from build123d import *

# Parameters (mm, degrees)
F0_R     = 38.1
F0_R_2   = 31.75
F1_DEPTH = 121.539
F2_DEPTH = 9.525
F3_R     = 5.08
F4_R     = 2.54


# Not quite as in the source:
# - a length typed as a fraction of an inch, garbled in the dataset ("3 / 203.2 mm" for 3/8 in), is restored


with BuildPart() as f1:
    # F0 (on Front) → F1 (new body)
    with BuildSketch(Plane.XZ):
        Circle(F0_R)
        Circle(F0_R_2, mode=Mode.SUBTRACT)
    extrude(amount=F1_DEPTH)

    # F0 (on Front) → F2 (join)
    with BuildSketch(Plane.XZ):
        Circle(F0_R_2)
    extrude(amount=F2_DEPTH)

    # F3
    f3_edges = [f1.edges().sort_by_distance(p)[0] for p in [
        (-38.1, -121.539, 0),
    ]]
    fillet(f3_edges, radius=F3_R)

    # F4
    f4_edges = [f1.edges().sort_by_distance(p)[0] for p in [
        (-31.75, -121.539, 0),
    ]]
    fillet(f4_edges, radius=F4_R)


solid = f1.part
Model file for the job. Use its own axes, mm. Give positions to 0.01 mm unless a question says otherwise; leave off trailing zeros. Order: outer loops, then holes, each group sorted by start corner. A loop starts at its lowest first (then second) coordinate and runs counter-clockwise, first axis right, second up. Notation, with made-up numbers: (-36.75, -35) - (13.25, -35) arc R17 cw to (13.25, -24) - close; hole circle Ø11 at (84, 48.25). An arc over 180 degrees is marked (long way). Write item = value, one per line. Start each with the question number.
1. Two-plate mould, pull along X, no slides. Class faces 1 (the flat face through (-1, 0, 1)), 2 (the cylindrical face through (-30.235, -57.414, -23.183)), 3 (the cylindrical face through (-6.883, -63.328, -30.995)): pulls with the +X half, pulls with the -X half, needs draft (parallel to the pull), parting line crosses it, or undercut.
2. Cut at A-A, the plane y = -12. List the corners of the cut face in (x, z), and give its area (3 significant figures).
3. Drop flat-ended pins along their axis: P1, Ø4, axis at x = 7, y = -67, coming from the -Z side; P2, Ø2, axis at y = -25.5, z = 19.5, coming from the -X side; P3, Ø1, axis at x = -17.5, y = -20.5, coming from the +Z side. Give the stop position or say it passes through.
4. Probe line 1 along Z through (x, y) = (0, -92); line 2 along Y through (x, z) = (-16, -16) (3 decimals); line 3 along Z through (x, y) = (4.5, -90). List the from-to ranges inside material, lowest first.
Taken from the geometry:
q1.face_1 = needs draft
q1.face_2 = parting line crosses it
q1.face_3 = undercut
q2.outline = circle Ø76.2 at (0, 0); hole circle Ø63.5 at (0, 0)
q2.area = 1,390 mm²
q3.P1 = -37.77
q3.P2 = -33.31
q3.P3 = 34.1
q4.line_1 = -38.1 to -31.75, 31.75 to 38.1
q4.line_2 = -9.525 to 0
q4.line_3 = -37.83 to -31.43, 31.43 to 37.83
